Geometry: final body of the model. Coordinates: model frame, mm. A direction names the side the tool comes from. Give positions to 0.01 mm unless a question says otherwise; leave off trailing zeros. Write each loop counter-clockwise with the first axis right and the second up, starting at its lowest first coordinate (ties: lowest second). Pieces come first, ordered by that corner, then holes. Notation, with made-up numbers: (2, 51.5) -> (52, 51.5) arc R28 cw to (52, 81.5) -> close; hole circle Ø1 at (18.5, 41). An arc over 180 degrees is marked (long way). Answer in a Markdown table with one row per item. Add a question column.
Item 1: Section query A-A on y = -11. Output: boundary loops of the cut face in (x, z), plus the area to 3 significant figures.
Item 2: Section query D-D on y = -8.5. Output: boundary loops of the cut face in (x, z), plus the area to 3 significant figures.
Item 3: Section query C-C on x = 10.25. Output: boundary loops of the cut face in (y, z).
Item 4: First-contact query: P1, Ø4, axis at y = -13, z = -2.5, coming from the +X side; P2, Ø3, axis at y = -11.5, z = -2, coming from the +X side; P3, Ø4, axis at y = -11.5, z = -2.5, coming from the +X side. Flat tips, straight axial feed; report the tip coordinate or a pass-through.
Item 5: Material intervals for probe 1 along Z at (x, y) = (-9, -10); probe 2 along X at (y, z) = (-10.75, -1.25); probe 3 along X at (y, z) = (-8.5, -1), sorted ascending. Write a range as from..to.
Item 6: Section query B-B on z = 0. Output: boundary loops of the cut face in (x, y), plus the area to 3 significant figures.
Item 7: Access query for faces 4 (the flat face through (-9, -10, 3)), 5 (the cylindrical face through (0, -12, 0)). Directions: +Z, -Z, +X, -X, +Y, -Y. A direction counts if a zero-diameter tool reaches every point of the face in a straight line with its end or side. Return the directions, or none.
Item 8: Draft query along Z for faces 1 (the flat face through (0, -13, 4)), 2 (the flat face through (-8.19, -10.674, 0.042)), 3 (the flat face through (10.761, -8.145, 0.056)). Return one class per face: +Z half, -Z half, draft (parallel to the pull), parting line (faces both ways), or undercut.
```python
from build123d import *

# Parameters (mm, degrees)
PAD001_DEPTH = 3
SKETCH004_R  = 10.5
POCKET_DEPTH = 5
PAD_DEPTH    = 4


with BuildPart() as body001:
    # Sketch001 → Pad001 (new body, symmetric)
    with BuildSketch(Plane.XY):
        with BuildLine():
            ThreePointArc((8.786596, -8.172865), (11.974307, -0.784838), (9.778199, 6.956064))
            Line((11.923388, 9.101253), (9.778199, 6.956064))
            Line((10.606602, 10.606602), (11.923388, 9.101253))
            Line((8.485281, 8.485281), (10.606602, 10.606602))
            ThreePointArc((8.485281, 8.485281), (0, 12), (-8.485281, 8.485281))
            Line((-8.485281, 8.485281), (-10.606602, 10.606602))
            Line((-10.606602, 10.606602), (-11.923388, 9.101253))
            Line((-11.923388, 9.101253), (-9.778199, 6.956064))
            ThreePointArc((-9.778199, 6.956064), (-11.974307, -0.784838), (-8.786596, -8.172865))
            Line((-8.786596, -8.172865), (-10.63343, -10.579705))
            Line((-10.63343, -10.579705), (-9.131421, -11.9003))
            Line((0, 0), (-9.131421, -11.9003))
            Line((0, 0), (9.131421, -11.9003))
            Line((9.131421, -11.9003), (10.63343, -10.579705))
            Line((10.63343, -10.579705), (8.786596, -8.172865))
        make_face()
    extrude(amount=PAD001_DEPTH, both=True)

    # Sketch004 → Pocket (cut)
    with BuildSketch(Plane.XY.offset(2.5)):
        Circle(SKETCH004_R)
    extrude(amount=-POCKET_DEPTH, mode=Mode.SUBTRACT)


with BuildPart() as body:
    # Sketch → Pad (new body, symmetric)
    with BuildSketch(Plane.XY):
        with BuildLine():
            ThreePointArc((-9.567984, -7.242492), (0, -12), (9.567984, -7.242492))
            Line((11.920113, -9.022938), (9.567984, -7.242492))
            ThreePointArc((-11.920113, -9.022938), (0, -14.95), (11.920113, -9.022938))
            Line((-11.920113, -9.022938), (-9.567984, -7.242492))
        make_face()
    extrude(amount=PAD_DEPTH, both=True)

    # Boolean: cut Body001
    add(body001.part, mode=Mode.SUBTRACT)


solid = body.part
```
Findings below:
| question | item | result |
|---|---|---|
| 1 | outline | (-10.12, -4) -> (-4.8, -4) -> (-4.8, 4) -> (-10.12, 4) -> (-10.12, 3) -> (-8.44, 3) -> (-8.44, -3) -> (-10.12, -3) -> close; (4.8, -4) -> (10.12, -4) -> (10.12, -3) -> (8.44, -3) -> (8.44, 3) -> (10.12, 3) -> (10.12, 4) -> (4.8, 4) -> close |
| 1 | area | 65.1 mm^2 |
| 2 | outline | (-11.23, -4) -> (-8.47, -4) -> (-8.47, -3) -> (-9.04, -3) -> (-9.04, 3) -> (-8.47, 3) -> (-8.47, 4) -> (-11.23, 4) -> close; (8.47, -4) -> (11.23, -4) -> (11.23, 4) -> (8.47, 4) -> (8.47, 3) -> (9.04, 3) -> (9.04, -3) -> (8.47, -3) -> close |
| 2 | area | 37.3 mm^2 |
| 3 | outline | (-10.88, -4) -> (-7.76, -4) -> (-7.76, 4) -> (-10.88, 4) -> (-10.88, 3) -> (-10.08, 3) -> (-10.08, -3) -> (-10.88, -3) -> close |
| 4 | P1 | stops at x = 10.05 |
| 4 | P2 | stops at x = 11.11 |
| 4 | P3 | stops at x = 11.54 |
| 5 | probe 1 | z = -4..-3, 3..4 |
| 5 | probe 2 | x = -8.25..-5.33, 5.33..8.25 |
| 5 | probe 3 | x = -11.23..-9.04, 9.04..11.23 |
| 6 | outline | (-11.92, -9.02) arc R14.95 ccw to (-10.6, -10.54) -> (-8.79, -8.17) arc R12 cw to (-9.57, -7.24) -> close; (-9.1, -11.86) arc R14.95 ccw to (9.1, -11.86) -> (7.31, -9.52) arc R12 cw to (-7.31, -9.52) -> close; (8.79, -8.17) -> (10.6, -10.54) arc R14.95 ccw to (11.92, -9.02) -> (9.57, -7.24) arc R12 cw to start |
| 6 | area | 61.6 mm^2 |
| 7 | face 4 | none |
| 7 | face 5 | +Z, -Z, +Y |
| 8 | face 1 | +Z half |
| 8 | face 2 | undercut |
| 8 | face 3 | draft |
